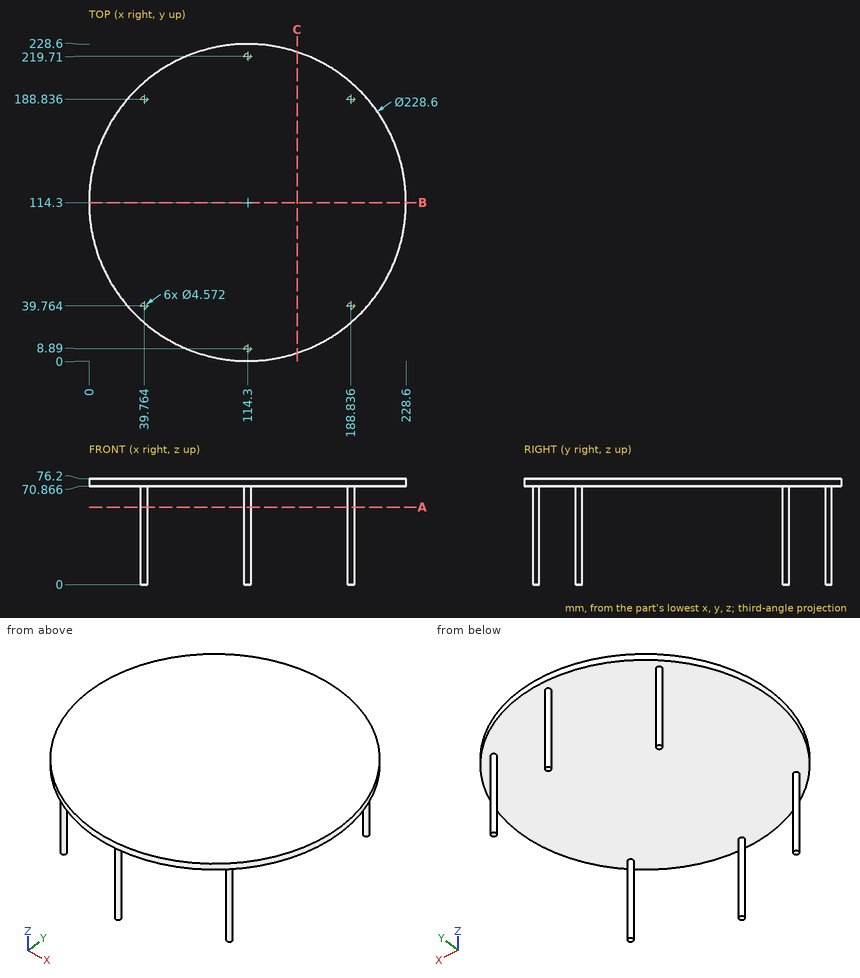
Input: dimensioned drawing with shaded views. Units: mm. Origin: part minimum x, y, z. Coordinates: 2 decimals unless noted, no trailing zeros. Write each loop counter-clockwise with the first axis right and the second up, starting at its lowest first coordinate (ties: lowest second). Pieces come first, ordered by that corner, then holes. Notation, with made-up numbers: M -8.5,-27 L 38.5,-27 A11 ccw 38.5,-22 Z; hole C 31,-23.5 d3. An arc over 180 degrees is marked long. Use one line per item in the form item = value.
Q1. Section C-C (x = 150). Return loops of the section in (y, z), plus the area to 3 significant figures.
Answer below:
outline = M 5.72,70.87 L 222.88,70.87 L 222.88,76.2 L 5.72,76.2 Z
area = 1,160 mm²
Q2. Material intervals for probe 1 along Z at (x, y) = (179, 96.5); probe 2 along X at (y, z) = (189.5, 17.5); probe 3 along Y at (x, z) = (87.5, 71.5), sorted ascending. Write a range as from..to.
Answer below:
probe_1 = 70.87..76.2
probe_2 = 37.58..41.95, 186.65..191.02
probe_3 = 3.19..225.41
Q3. First-contact query: pin 1 (1 mm diameter, centred on x = 139, y = 87, fed in from -Z). Flat tip, straight axial feed; report the tip coordinate or a pass-through.
Answer below:
pin_1 = 70.87
Q4. Section A-A (z = 56). Return loops of the section in (x, y).
Answer below:
outline = C 39.76,39.76 d4.57; C 39.76,188.84 d4.57; C 114.3,8.89 d4.57; C 114.3,219.71 d4.57; C 188.84,39.76 d4.57; C 188.84,188.84 d4.57
Q5. Section B-B (y = 114.3). Return loops of the section in (x, z), plus the area to 3 significant figures.
Answer below:
outline = M 0,70.87 L 228.6,70.87 L 228.6,76.2 L 0,76.2 Z
area = 1,220 mm²
